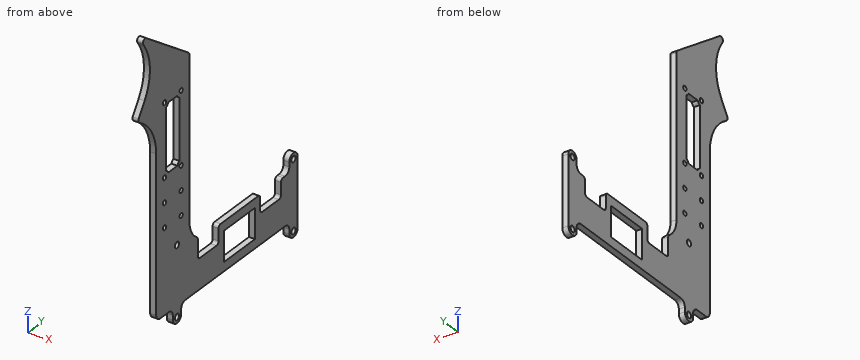
```python
from build123d import *

# Parameters (mm, degrees)
SKETCH2_R           = 2.4892
SKETCH2_R_2         = 3.175
SKETCH2_R_3         = 6.35
BOSS_EXTRUDE1_DEPTH = 6.35
FILLET1_R           = 25.4
FILLET2_R           = 6.35
FILLET3_R           = 12.7
SKETCH3_W           = 19.05
SKETCH3_H           = 31.75
CUT_EXTRUDE1_DEPTH  = 410.639602463
FILLET4_R           = 3.175
BOSS_EXTRUDE2_START = -6.35
BOSS_EXTRUDE2_DEPTH = 6.35
FILLET5_R           = 50.8
FILLET6_R           = 3.1496
SKETCH5_W           = 31.75
SKETCH5_H           = 47.625
CUT_EXTRUDE2_DEPTH  = 410.639602463


with BuildPart() as part:
    # Sketch2 → Boss-Extrude1 (new body)
    # profile 1 of 8: a face of its own
    with BuildSketch(Plane(origin=(228.6, 0, 0), x_dir=(0, 0, -1), z_dir=(1, 0, 0))):
        Polygon((190.5, 152.4), (12.7, 152.4), (12.7, 101.6), (241.3, 101.6), (241.3, 127), (241.3, 139.7), (241.3, 152.4), align=None)
        with Locations((25.4, 114.3)):
            Circle(SKETCH2_R, mode=Mode.SUBTRACT)
        with Locations((25.4, 139.7)):
            Circle(SKETCH2_R, mode=Mode.SUBTRACT)
        with Locations((101.6, 114.3)):
            Circle(SKETCH2_R, mode=Mode.SUBTRACT)
        with Locations((127, 114.3)):
            Circle(SKETCH2_R, mode=Mode.SUBTRACT)
        with Locations((101.6, 139.7)):
            Circle(SKETCH2_R, mode=Mode.SUBTRACT)
        with Locations((127, 139.7)):
            Circle(SKETCH2_R, mode=Mode.SUBTRACT)
        with Locations((152.4, 114.3)):
            Circle(SKETCH2_R, mode=Mode.SUBTRACT)
        with Locations((152.4, 139.7)):
            Circle(SKETCH2_R, mode=Mode.SUBTRACT)
        with Locations((179.3875, 133.35)):
            Circle(SKETCH2_R_2, mode=Mode.SUBTRACT)
    # profile 2 of 8: a face of its own
    with BuildSketch(Plane(origin=(228.6, 0, 0), x_dir=(0, 0, -1), z_dir=(1, 0, 0))):
        Polygon((190.5, 304.8), (190.5, 152.4), (241.3, 152.4), (241.3, 304.8), (241.3, 317.5), (190.5, 317.5), align=None)
    # profile 3 of 8: a face of its own
    with BuildSketch(Plane(origin=(228.6, 0, 0), x_dir=(0, 0, -1), z_dir=(1, 0, 0))):
        with BuildLine():
            Line((179.3875, 304.8), (190.5, 304.8))
            Line((190.5, 304.8), (190.5, 317.5))
            Line((190.5, 317.5), (179.3875, 317.5))
            ThreePointArc((179.3875, 317.5), (183.877628061, 315.640128061), (185.7375, 311.15))
            ThreePointArc((185.7375, 311.15), (183.877628061, 306.659871939), (179.3875, 304.8))
        make_face()
    # profile 4 of 8: a face of its own
    with BuildSketch(Plane(origin=(228.6, 0, 0), x_dir=(0, 0, -1), z_dir=(1, 0, 0))):
        with Locations((179.3875, 311.15)):
            Circle(SKETCH2_R_3)
        with Locations((179.3875, 311.15)):
            Circle(SKETCH2_R_2, mode=Mode.SUBTRACT)
    # profile 5 of 8: a face of its own
    with BuildSketch(Plane(origin=(228.6, 0, 0), x_dir=(0, 0, -1), z_dir=(1, 0, 0))):
        with Locations((252.4125, 311.15)):
            Circle(SKETCH2_R_3)
        with Locations((252.4125, 311.15)):
            Circle(SKETCH2_R_2, mode=Mode.SUBTRACT)
    # profile 6 of 8: a face of its own
    with BuildSketch(Plane(origin=(228.6, 0, 0), x_dir=(0, 0, -1), z_dir=(1, 0, 0))):
        with BuildLine():
            Line((241.3, 317.5), (241.3, 304.8))
            Line((241.3, 304.8), (252.4125, 304.8))
            ThreePointArc((252.4125, 304.8), (246.0625, 311.15), (252.4125, 317.5))
            Line((252.4125, 317.5), (241.3, 317.5))
        make_face()
    # profile 7 of 8: a face of its own
    with BuildSketch(Plane(origin=(228.6, 0, 0), x_dir=(0, 0, -1), z_dir=(1, 0, 0))):
        with BuildLine():
            Line((252.4125, 139.7), (241.3, 139.7))
            Line((241.3, 139.7), (241.3, 127))
            Line((241.3, 127), (252.4125, 127))
            ThreePointArc((252.4125, 127), (246.0625, 133.35), (252.4125, 139.7))
        make_face()
    # profile 8 of 8: a face of its own
    with BuildSketch(Plane(origin=(228.6, 0, 0), x_dir=(0, 0, -1), z_dir=(1, 0, 0))):
        with Locations((252.4125, 133.35)):
            Circle(SKETCH2_R_3)
        with Locations((252.4125, 133.35)):
            Circle(SKETCH2_R_2, mode=Mode.SUBTRACT)
    extrude(amount=-BOSS_EXTRUDE1_DEPTH)

    # Fillet1
    fillet1_edges = [part.edges().sort_by_distance(p)[0] for p in [
        (225.425, 152.4, -190.5),
    ]]
    fillet(fillet1_edges, radius=FILLET1_R)

    # Fillet2
    fillet2_edges = [part.edges().sort_by_distance(p)[0] for p in [
        (225.425, 139.7, -241.3),
        (225.425, 127, -241.3),
        (225.425, 101.6, -241.3),
        (225.425, 304.8, -190.5),
        (225.425, 304.8, -241.3),
    ]]
    fillet(fillet2_edges, radius=FILLET2_R)

    # Fillet3
    fillet3_edges = [part.edges().sort_by_distance(p)[0] for p in [
        (225.425, 101.6, -12.7),
        (225.425, 152.4, -12.7),
    ]]
    fillet(fillet3_edges, radius=FILLET3_R)

    # Sketch3 → Cut-Extrude1 (cut, through all)
    with BuildSketch(Plane(origin=(228.6, 0, 0), x_dir=(0, 0, -1), z_dir=(1, 0, 0))):
        with BuildLine():
            Line((190.5, 177.8), (190.5, 190.18276047))
            Line((190.5, 190.18276047), (98.023677914, 190.18276047))
            Line((98.023677914, 190.18276047), (98.023677914, 165.1))
            Line((98.023677914, 165.1), (187.097045256, 165.1))
            ThreePointArc((187.097045256, 165.1), (189.634515988, 171.225996254), (190.5, 177.8))
        make_face()
        with Locations((200.025, 276.225)):
            Rectangle(SKETCH3_W, SKETCH3_H)
        with BuildLine():
            Line((190.5, 165.1), (190.5, 177.8))
            ThreePointArc((190.5, 177.8), (189.634515988, 171.225996254), (187.097045256, 165.1))
            Line((187.097045256, 165.1), (190.5, 165.1))
        make_face()
        Polygon((209.55, 196.85), (190.5, 196.85), (190.5, 190.18276047), (190.5, 177.8), (190.5, 165.1), (209.55, 165.1), align=None)
    extrude(amount=-CUT_EXTRUDE1_DEPTH, mode=Mode.SUBTRACT)

    # Fillet4
    fillet4_edges = [part.edges().sort_by_distance(p)[0] for p in [
        (225.425, 165.1, -187.097045256),
        (225.425, 292.1, -190.5),
        (225.425, 292.1, -209.55),
        (225.425, 260.35, -209.55),
        (225.425, 260.35, -190.5),
        (225.425, 165.1, -209.55),
        (225.425, 196.85, -190.5),
        (225.425, 196.85, -209.55),
    ]]
    fillet(fillet4_edges, radius=FILLET4_R)

    # Sketch4 → Boss-Extrude2 (add)
    with BuildSketch(Plane(origin=(228.6, 0, 0), x_dir=(0, 0, -1), z_dir=(1, 0, 0)).offset(BOSS_EXTRUDE2_START)):
        with BuildLine():
            Line((-6.35, 152.4), (-63.5, 73.025))
            Line((-63.5, 73.025), (-19.05, 101.6))
            Line((-19.05, 101.6), (25.4, 73.025))
            Line((25.4, 73.025), (25.4, 101.6))
            ThreePointArc((25.4, 101.6), (16.419743879, 105.319743879), (12.7, 114.3))
            Line((12.7, 114.3), (12.7, 139.7))
            ThreePointArc((12.7, 139.7), (16.419743879, 148.680256121), (25.4, 152.4))
            Line((25.4, 152.4), (-6.35, 152.4))
        make_face()
    extrude(amount=BOSS_EXTRUDE2_DEPTH)

    # Fillet5
    # the kernel refuses this fillet: 50.8 mm, written as the material it adds along each edge
    with BuildSketch(Plane(origin=(222.25, 101.6, 19.05), x_dir=(0, -0.5407575913134988, -0.8411784753765537), z_dir=(1, 0, 0))) as fillet5_piece_1:
        with BuildLine():
            CenterArc((FILLET5_R * 0.642857142857, -FILLET5_R), FILLET5_R, 90, 65.470452544)
            Line((-FILLET5_R * 0.266890149562, -FILLET5_R * 0.584837545126), (-FILLET5_R * 0.28508509541, -FILLET5_R * 0.576534296029))
            Line((-FILLET5_R * 0.28508509541, -FILLET5_R * 0.576534296029), (-FILLET5_R * 0.0128571428571, FILLET5_R * 0.02))
            Line((-FILLET5_R * 0.0128571428571, FILLET5_R * 0.02), (FILLET5_R * 0.642857142857, FILLET5_R * 0.02))
            Line((FILLET5_R * 0.642857142857, FILLET5_R * 0.02), (FILLET5_R * 0.642857142857, 0))
        make_face()
    extrude(amount=6.35)
    with BuildSketch(Plane(origin=(228.6, 101.6, -25.4), x_dir=(0, 0, -1), z_dir=(-1, 0, 0))) as fillet5_piece_2_section:
        with BuildLine():
            CenterArc((45.68029526, 50.8), FILLET5_R, 205.944479772, 64.055520228)
            Line((0, 28.575), (-0.913605905, 28.1305))
            ThreePointArc((-0.913605905, 28.1305), (-1.016, 14.2875), (-1.016, 0))
            Line((-1.016, 0), (0, -1.016))
            Line((0, -1.016), (45.68029526, -1.016))
            Line((45.68029526, -1.016), (45.68029526, 0))
        make_face()
    fillet5_piece_2 = extrude(amount=6.35, mode=Mode.PRIVATE)
    fillet5_piece_2 = split(fillet5_piece_2, bisect_by=Plane(origin=(225.425, 74.109510014, -23.712984423), z_dir=(0, 0.8411784753765535, -0.5407575913134988)), keep=Keep.TOP, mode=Mode.PRIVATE)
    add(fillet5_piece_2)

    # Fillet6
    fillet6_edges = [part.edges().sort_by_distance(p)[0] for p in [
        (225.425, 73.025, -25.4),
        (225.425, 73.025, 63.5),
        (225.425, 152.4, 6.35),
    ]]
    fillet(fillet6_edges, radius=FILLET6_R)

    # Sketch5 → Cut-Extrude2 (cut, through all)
    with BuildSketch(Plane(origin=(228.6, 0, 0), x_dir=(0, 0, -1), z_dir=(1, 0, 0))):
        with Locations((215.9, 228.6)):
            Rectangle(SKETCH5_W, SKETCH5_H)
        with BuildLine():
            ThreePointArc((99.06, 133.880128867), (97.109871939, 135.209871939), (95.780128867, 137.16))
            Line((95.780128867, 137.16), (31.219871133, 137.16))
            ThreePointArc((31.219871133, 137.16), (29.890128061, 135.209871939), (27.94, 133.880128867))
            Line((27.94, 133.880128867), (27.94, 120.119871133))
            ThreePointArc((27.94, 120.119871133), (29.890128061, 118.790128061), (31.219871133, 116.84))
            Line((31.219871133, 116.84), (95.780128867, 116.84))
            ThreePointArc((95.780128867, 116.84), (97.109871939, 118.790128061), (99.06, 120.119871133))
            Line((99.06, 120.119871133), (99.06, 133.880128867))
        make_face()
    extrude(amount=-CUT_EXTRUDE2_DEPTH, mode=Mode.SUBTRACT)


solid = part.part
```
The model under review builds one solid part; all positions refer to its coordinate system, in mm. Give positions to 0.01 mm unless a question says otherwise; leave off trailing zeros. Write each loop counter-clockwise with the first axis right and the second up, starting at its lowest first coordinate (ties: lowest second). Pieces come first, ordered by that corner, then holes. Notation, with made-up numbers: M 23,83 L 34,83 A27 cw 34,118 Z; hole C 58,-36 d5. An arc over 180 degrees is marked long. Write item = value, one per line. Start each with the question number.
Q1. For line 1 (Y direction, x = 223.5, z = -152.4); line 2 (Y direction, x = 225.25, z = -181.5); line 3 (Y direction, x = 222.75, z = -153), list the stretches that pass through material, from the lowest coordinate up.
Q2. We need section D-D (x = 227). Give the number of separate pieces and of enclosed holes in the cut face, plus the area to 3 significant figures.
Q3. Clearance check with flat-ended pins moving along their axes: pin 1 (3 mm diameter, centred on x = 224.5, z = -161, fed in from -Y); pin 2 (1.9 mm diameter, centred on x = 224.5, y = 129, fed in from -Z); pin 3 (1.9 mm diameter, centred on x = 226.5, y = 282.5, fed in from +Z). State where each tip first meets the part, or that it passes through.
Q4. We need section A-A (z = -213.5). State the section outline as (x, y) points, plus the area to 3 significant figures.
Q5. We need section B-B (y = 311.15). State the section outline as (x, z) points, plus the area to 3 significant figures.
Q6. We need section C-C (y = 226.5). State the section outline as (x, z) points (3 decimals).
Result set:
q1.line_1 = 101.6 to 111.81, 116.79 to 137.21, 142.19 to 152.4
q1.line_2 = 101.6 to 130.98, 135.72 to 158.4, 304.8 to 308.78, 313.52 to 317.5
q1.line_3 = 101.6 to 111.88, 116.72 to 137.28, 142.12 to 152.4
q2.separate_pieces = 1
q2.enclosed_holes = 14
q2.area = 19,700 mm2
q3.pin_1 = 101.6
q3.pin_2 = -257.78
q3.pin_3 = -209.55
q4.outline = M 222.25,101.6 L 228.6,101.6 L 228.6,204.79 L 222.25,204.79 Z; M 222.25,252.41 L 228.6,252.41 L 228.6,317.5 L 222.25,317.5 Z
q4.area = 1,070 mm2
q5.outline = M 222.25,-258.76 L 228.6,-258.76 L 228.6,-255.59 L 222.25,-255.59 Z; M 222.25,-249.24 L 228.6,-249.24 L 228.6,-182.56 L 222.25,-182.56 Z; M 222.25,-176.21 L 228.6,-176.21 L 228.6,-173.04 L 222.25,-173.04 Z
q5.area = 464 mm2
q6.outline = M 222.25,-241.3 L 228.6,-241.3 L 228.6,-231.775 L 222.25,-231.775 Z; M 222.25,-200.025 L 228.6,-200.025 L 228.6,-190.5 L 222.25,-190.5 Z
